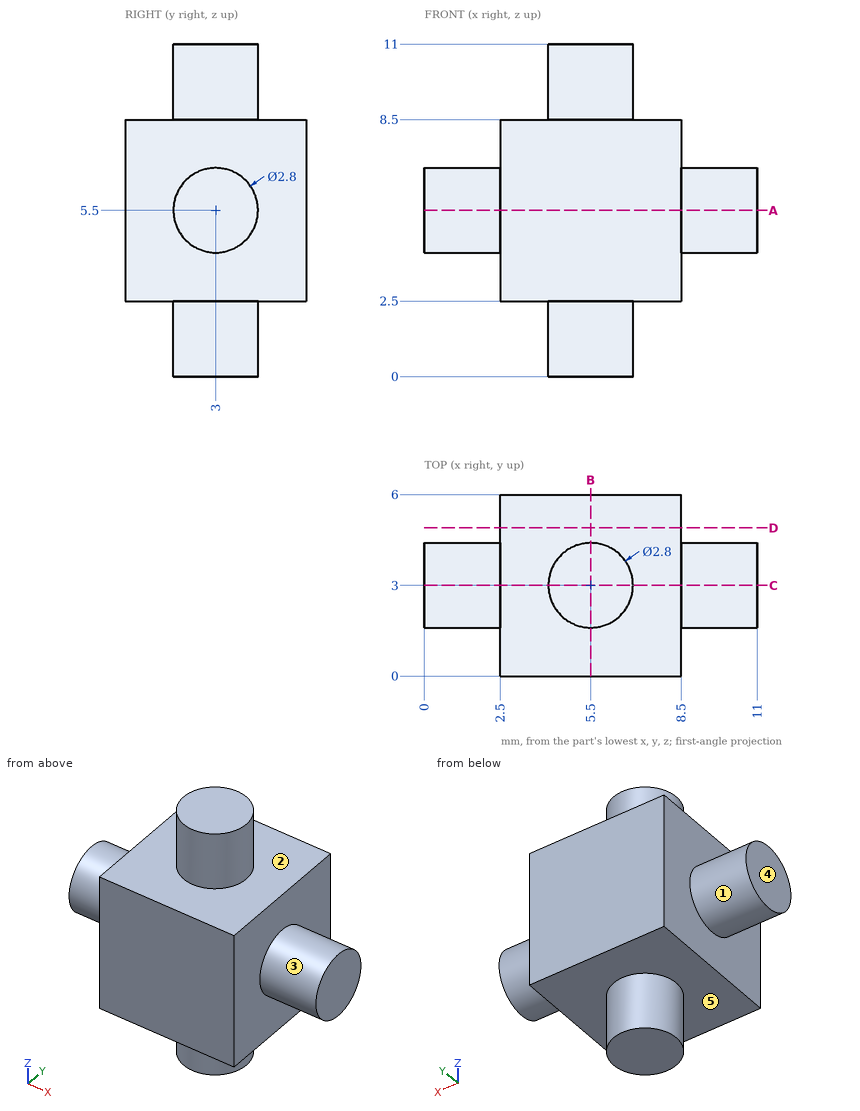
Verification items for this drawing (mm, ordinates from the low corner). A direction names the side the tool comes from. Coordinates: 2 decimals unless noted, no trailing zeros. Order: outer loops, then holes, each group sorted by start corner. A loop starts at its lowest first (then second) coordinate and runs counter-clockwise, first axis right, second up. Notation, with made-up numbers: (58, 50.5) -> (86, 50.5) arc R20 ccw to (86, 63.5) -> close; hole circle Ø2 at (-31.5, -31). An arc over 180 degrees is marked (long way). Answer as CSV lines item,"result". Start each with the question number.
1) Cross-section at D-D, the plane y = 4.9. Record the boundary of the cut face in (x, z), then the cut area to 3 significant figures.
2) Cross-section at C-C, the plane y = 3. Record the boundary of the cut face in (x, z).
3) Cross-section at B-B, the plane x = 5.5. Record the boundary of the cut face in (y, z), then the cut area to 3 significant figures.
4) Gauge pin test, flat end, axial feed: pin 1 Ø1 at (y, z) = (5.5, 8) entering from -X. Record the tip position at first contact, or that the pin passes through.
5) Material ranges on L1, parallel to Z at x = 5, y = 4.55; L2, parallel to Y at x = 2, z = 4.75, recorded low to high. Write a range as [from, to].
6) Set-up check for the marked faces 1, 2, 3, 4 and 5: record each of +Z, -Z, +X, -X, +Y, -Y from which the full face is reachable in a straight line by a thin tool's end or side.
7) Cross-section at A-A, the plane z = 5.5. Record the boundary of the cut face in (x, y), then the cut area to 3 significant figures.
Conclusion:
1,outline,"(2.5, 2.5) -> (8.5, 2.5) -> (8.5, 8.5) -> (2.5, 8.5) -> close"
1,area,"36.0 mm²"
2,outline,"(0, 4.1) -> (2.5, 4.1) -> (2.5, 2.5) -> (4.1, 2.5) -> (4.1, 0) -> (6.9, 0) -> (6.9, 2.5) -> (8.5, 2.5) -> (8.5, 4.1) -> (11, 4.1) -> (11, 6.9) -> (8.5, 6.9) -> (8.5, 8.5) -> (6.9, 8.5) -> (6.9, 11) -> (4.1, 11) -> (4.1, 8.5) -> (2.5, 8.5) -> (2.5, 6.9) -> (0, 6.9) -> close"
3,outline,"(0, 2.5) -> (1.6, 2.5) -> (1.6, 0) -> (4.4, 0) -> (4.4, 2.5) -> (6, 2.5) -> (6, 8.5) -> (4.4, 8.5) -> (4.4, 11) -> (1.6, 11) -> (1.6, 8.5) -> (0, 8.5) -> close"
3,area,"50.0 mm²"
4,pin 1,"stops at x = 2.5"
5,L1,"z = [2.5, 8.5]"
5,L2,"y = [1.82, 4.18]"
6,face 1,"-X"
6,face 2,"+Z"
6,face 3,"+X"
6,face 4,"+Z, -Z, -X, +Y, -Y"
6,face 5,"-Z"
7,outline,"(0, 1.6) -> (2.5, 1.6) -> (2.5, 0) -> (8.5, 0) -> (8.5, 1.6) -> (11, 1.6) -> (11, 4.4) -> (8.5, 4.4) -> (8.5, 6) -> (2.5, 6) -> (2.5, 4.4) -> (0, 4.4) -> close"
7,area,"50.0 mm²"
